```python
from build123d import *

# Parameters (mm, degrees)
F0_R     = 3.175
F0_R_2   = 1.5875
F1_DEPTH = 6.35


with BuildPart() as f1:
    # F0 (on Front) → F1 (new body)
    with BuildSketch(Plane.XZ):
        with BuildLine():
            ThreePointArc((0.34024, -73.018883), (6.854439, -70.113772), (9.525014, -63.499961))
            ThreePointArc((9.525014, -63.499961), (0.517595, -53.989034), (-9.468736, -62.46633))
            ThreePointArc((-9.468736, -62.46633), (-6.976488, -69.98487), (0.34024, -73.018883))
        make_face()
        with Locations((1.4e-05, -63.499961)):
            Circle(F0_R, mode=Mode.SUBTRACT)
        with BuildLine():
            ThreePointArc((-9.468736, -62.46633), (0.517595, -53.989034), (9.525014, -63.499961))
            ThreePointArc((9.525014, -63.499961), (6.854439, -70.113772), (0.34024, -73.018883))
            Line((0.34024, -73.018883), (44.669469, -71.434466))
            ThreePointArc((44.669469, -71.434466), (36.512502, -63.495435), (44.678596, -55.565793))
            Line((44.678596, -55.565793), (18.853, -54.642728))
            ThreePointArc((18.853, -54.642728), (13.139918, -51.916888), (11.228697, -45.882259))
            Line((11.228697, -45.882259), (15.791295, -1.62808))
            ThreePointArc((15.791295, -1.62808), (0.006474, -15.874999), (-15.789961, -1.640958))
            Line((-15.789961, -1.640958), (-9.468736, -62.46633))
        make_face()
        with BuildLine():
            ThreePointArc((-15.74798, 2.004183), (-15.873947, 0.182821), (-15.789961, -1.640958))
            ThreePointArc((-15.789961, -1.640958), (0.006474, -15.874999), (15.791295, -1.62808))
            ThreePointArc((15.791295, -1.62808), (15.85406, -0.815115), (15.875, 0))
            ThreePointArc((15.875, 0), (15.842921, 1.008708), (15.746812, 2.013339))
            ThreePointArc((15.746812, 2.013339), (-0.004615, 15.874999), (-15.74798, 2.004183))
        make_face()
        Circle(F0_R, mode=Mode.SUBTRACT)
        with BuildLine():
            ThreePointArc((44.678596, -55.565793), (36.512502, -63.495435), (44.669469, -71.434466))
            ThreePointArc((44.669469, -71.434466), (50.139726, -69.034523), (52.387501, -63.500001))
            ThreePointArc((52.387501, -63.500001), (50.142908, -57.968752), (44.678596, -55.565793))
        make_face()
        with Locations((44.450001, -63.500001)):
            Circle(F0_R, mode=Mode.SUBTRACT)
        with BuildLine():
            Line((-9.468391, 51.346407), (-15.74798, 2.004183))
            ThreePointArc((-15.74798, 2.004183), (-0.004615, 15.874999), (15.746812, 2.013339))
            Line((15.746812, 2.013339), (9.558254, 50.415554))
            ThreePointArc((9.558254, 50.415554), (-0.424197, 41.291985), (-9.468391, 51.346407))
        make_face()
        with Locations((-1.569617, 36.038321)):
            Circle(F0_R_2, mode=Mode.SUBTRACT)
        with BuildLine():
            ThreePointArc((9.566244, 50.805606), (0.311753, 60.326764), (-9.468391, 51.346407))
            ThreePointArc((-9.468391, 51.346407), (-0.424197, 41.291985), (9.558254, 50.415554))
            ThreePointArc((9.558254, 50.415554), (9.564246, 50.610539), (9.566244, 50.805606))
        make_face()
        with Locations((0.041244, 50.805606)):
            Circle(F0_R, mode=Mode.SUBTRACT)
    extrude(amount=F1_DEPTH)


solid = f1.part
```
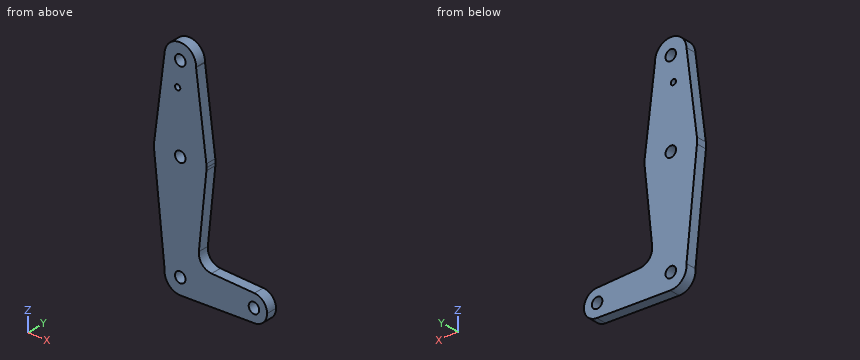
Input: part model. Units: mm. Frame: model coordinates. Give positions to 0.01 mm unless a question says otherwise; leave off trailing zeros. Loops run counter-clockwise (first coordinate to the right, second up) from the corner with the lowest first, then second, coordinate; pieces in that order, holes last.
1) Section query A-A on y = -1.25. Count the separate pieces of the cut face and the enclosed holes in it, and give its area (3 significant figures).
A:
separate pieces: 1
enclosed holes: 5
area: 3,780 mm2
2) Section query B-B on z = -11. Return the cut outline in (x, y), and give its area (3 significant figures).
A:
outline: (-14.82, -6.35) - (14.83, -6.35) - (14.83, 0) - (-14.82, 0) - close
area: 188 mm2
3) Line query: L1, parallel to X at y = -3.5, z = 51; L2, parallel to Z at x = 44.45, y = -4 (3 decimals); L3, parallel to Z at x = 5, y = -0.25. Output: solid intervals per line, ascending.
A:
L1: x = -9.51 to -3.13, 3.21 to 9.56
L2: z = -71.442 to -66.675, -60.325 to -55.558
L3: z = -72.85 to 58.94
4) Contact query for a flat-ended pin moving along its axis: pin 1 (1 mm diameter, centred on x = 30, y = -1.5, fed in from +Z). Output: stop coordinate, or through.
A:
pin 1: stops at z = -55.02
5) Section query C-C on x = -5. Return the cut outline in (y, z), and give its area (3 significant figures).
A:
outline: (-6.35, -71.61) - (0, -71.61) - (0, 58.89) - (-6.35, 58.89) - close
area: 829 mm2
